```python
from build123d import *

# Parameters (mm, degrees)
EXTRUDE_1_DEPTH       = 2
SKETCH_2_R            = 1.6
CUT_EXTRUDE_1_DEPTH   = 2
CUT_EXTRUDE_2_DEPTH   = 10
EXTRUDE_START         = -2
EXTRUDE_1_2_OUTLINE_R = 16.5
EXTRUDE_1_2_DEPTH     = 2
SKETCH_5_R            = 1.6
CUT_EXTRUDE_3_DEPTH   = 2
FILLET_1_R            = 2
FILLET_2_R            = 2
SKETCH_6_W            = 33
SKETCH_6_H            = 4
EXTRUDE_2_DEPTH       = 2
FILLET_3_R            = 2


# Read off the part's stored shape, not the designer's step: 拉伸-薄壁1
with BuildPart() as part:
    # 草图1 → Extrude 1 (new body)
    with BuildSketch(Plane(origin=(0, 0, 0), x_dir=(1, 0, 0), z_dir=(0, 1, 0))):
        Polygon((0, 0), (121, 0), (121, -82), (-39.6, -82), (-39.6, 29), (0, 29), align=None)
    extrude(amount=EXTRUDE_1_DEPTH)

    # 草图2 → 切除-拉伸1 (cut)
    with BuildSketch(Plane(origin=(0, 2, 0), x_dir=(1, 0, 0), z_dir=(0, 1, 0))):
        with Locations(Location((-34.6, -75, 0), (0, 0, 270))):
            Circle(SKETCH_2_R)
        with Locations(Location((-34.6, 22, 0), (0, 0, 270))):
            Circle(SKETCH_2_R)
        with Locations(Location((116, -75, 0), (0, 0, 270))):
            Circle(SKETCH_2_R)
        with Locations(Location((116, -7, 0), (0, 0, 270))):
            Circle(SKETCH_2_R)
        with Locations(Location((5, -7, 0), (0, 0, 270))):
            Circle(SKETCH_2_R)
    extrude(amount=-CUT_EXTRUDE_1_DEPTH, mode=Mode.SUBTRACT)

    # 草图3 → 切除-拉伸2 (cut)
    with BuildSketch(Plane(origin=(0, 2, 0), x_dir=(1, 0, 0), z_dir=(0, 1, 0))):
        with BuildLine():
            Line((-8, 24), (-30.017424305, 24))
            ThreePointArc((-30.017424305, 24), (-30.162628331, 19.695714283), (-33.6, 17.101020514))
            Line((-33.6, 17.101020514), (-33.6, -70.101020514))
            ThreePointArc((-33.6, -70.101020514), (-30.428791604, -72.243005166), (-29.701020514, -76))
            Line((-29.701020514, -76), (-8, -76))
            Line((-8, -76), (-8, 24))
        make_face()
        with BuildLine():
            ThreePointArc((10, -7), (5, -12), (0, -7))
            Line((0, -7), (0, -75))
            Line((0, -75), (111, -75))
            ThreePointArc((111, -75), (111.527864045, -72.763932023), (113, -71))
            Line((113, -71), (113, -11))
            ThreePointArc((113, -11), (111.527864045, -9.236067977), (111, -7))
            Line((111, -7), (10, -7))
        make_face()
    extrude(amount=-CUT_EXTRUDE_2_DEPTH, mode=Mode.SUBTRACT)

    # Extrude 1 2 outline → Extrude 1 2 (add)
    # profile 1 of 4: a face of its own
    with BuildSketch(Plane(origin=(0, 2, 0), x_dir=(1, 0, 0), z_dir=(0, 1, 0)).offset(EXTRUDE_START)):
        with BuildLine():
            Line((87.508781443, -59.891378935), (111.047620543, -74.311568655))
            ThreePointArc((111.047620543, -74.311568655), (111.692830803, -72.460650968), (113, -71))
            Line((113, -71), (113, -70.81670339))
            Line((113, -70.81670339), (91.231047509, -57.480768531))
            Line((91.231047509, -57.480768531), (113, -43.382780251))
            Line((113, -43.382780251), (113, -38.617219749))
            Line((113, -38.617219749), (91.231047509, -24.519231469))
            Line((91.231047509, -24.519231469), (113, -11.18329661))
            Line((113, -11.18329661), (113, -11))
            ThreePointArc((113, -11), (111.692830803, -9.539349032), (111.047620543, -7.688431345))
            Line((111.047620543, -7.688431345), (87.508781443, -22.108621065))
            Line((87.508781443, -22.108621065), (64.179293034, -7))
            Line((64.179293034, -7), (56.417693677, -7))
            Line((56.417693677, -7), (31.597528439, -20.948522613))
            Line((31.597528439, -20.948522613), (9.952379457, -7.688431345))
            ThreePointArc((9.952379457, -7.688431345), (9.263558208, -9.611909533), (7.86285183, -11.099277912))
            Line((7.86285183, -11.099277912), (27.603885339, -23.192884025))
            Line((27.603885339, -23.192884025), (0, -38.705811323))
            Line((0, -38.705811323), (0, -43.294188677))
            Line((0, -43.294188677), (27.603885339, -58.807115975))
            Line((27.603885339, -58.807115975), (1.171383475, -75))
            Line((1.171383475, -75), (8.828616525, -75))
            Line((8.828616525, -75), (31.597528439, -61.051477387))
            Line((31.597528439, -61.051477387), (56.417693677, -75))
            Line((56.417693677, -75), (64.179293034, -75))
            Line((64.179293034, -75), (87.508781443, -59.891378935))
        make_face()
        with BuildLine():
            Line((35.503873282, -58.658401266), (44.147565445, -53.363166428))
            ThreePointArc((44.147565445, -53.363166428), (50.482041032, -58.885482887), (58.5, -61.402205763))
            Line((58.5, -61.402205763), (58.5, -71.581844381))
            Line((58.5, -71.581844381), (35.503873282, -58.658401266))
        make_face(mode=Mode.SUBTRACT)
        with BuildLine():
            Line((76.852434555, -53.363166428), (83.727285824, -57.574787025))
            Line((83.727285824, -57.574787025), (62.5, -71.321981654))
            Line((62.5, -71.321981654), (62.5, -61.402205763))
            ThreePointArc((62.5, -61.402205763), (70.517958968, -58.885482887), (76.852434555, -53.363166428))
        make_face(mode=Mode.SUBTRACT)
        with BuildLine():
            Line((31.510230182, -25.585960145), (42.058037819, -32.047680139))
            ThreePointArc((42.058037819, -32.047680139), (40, -41), (42.058037819, -49.952319861))
            Line((42.058037819, -49.952319861), (31.510230182, -56.414039855))
            Line((31.510230182, -56.414039855), (4.082306323, -41))
            Line((4.082306323, -41), (31.510230182, -25.585960145))
        make_face(mode=Mode.SUBTRACT)
        with BuildLine():
            Line((58.5, -10.418155619), (58.5, -20.597794237))
            ThreePointArc((58.5, -20.597794237), (50.482041032, -23.114517113), (44.147565445, -28.636833572))
            Line((44.147565445, -28.636833572), (35.503873282, -23.341598734))
            Line((35.503873282, -23.341598734), (58.5, -10.418155619))
        make_face(mode=Mode.SUBTRACT)
        with Locations((60.5, -41)):
            Circle(EXTRUDE_1_2_OUTLINE_R, mode=Mode.SUBTRACT)
        with BuildLine():
            Line((87.449551891, -26.83582338), (109.320706966, -41))
            Line((109.320706966, -41), (87.449551891, -55.16417662))
            Line((87.449551891, -55.16417662), (78.941962181, -49.952319861))
            ThreePointArc((78.941962181, -49.952319861), (81, -41), (78.941962181, -32.047680139))
            Line((78.941962181, -32.047680139), (87.449551891, -26.83582338))
        make_face(mode=Mode.SUBTRACT)
        with BuildLine():
            ThreePointArc((76.852434555, -28.636833572), (70.517958968, -23.114517113), (62.5, -20.597794237))
            Line((62.5, -20.597794237), (62.5, -10.678018346))
            Line((62.5, -10.678018346), (83.727285824, -24.425212975))
            Line((83.727285824, -24.425212975), (76.852434555, -28.636833572))
        make_face(mode=Mode.SUBTRACT)
    # profile 2 of 4: a face of its own
    with BuildSketch(Plane(origin=(0, 2, 0), x_dir=(1, 0, 0), z_dir=(0, 1, 0)).offset(EXTRUDE_START)):
        with BuildLine():
            Line((115.16418895, -76.364338627), (116.83581105, -73.635661373))
            ThreePointArc((116.83581105, -73.635661373), (114.635661373, -74.16418895), (115.16418895, -76.364338627))
        make_face()
    # profile 3 of 4: a face of its own
    with BuildSketch(Plane(origin=(0, 2, 0), x_dir=(1, 0, 0), z_dir=(0, 1, 0)).offset(EXTRUDE_START)):
        with BuildLine():
            Line((116.83581105, -8.364338627), (115.16418895, -5.635661373))
            ThreePointArc((115.16418895, -5.635661373), (114.635661373, -7.83581105), (116.83581105, -8.364338627))
        make_face()
    # profile 4 of 4: a face of its own
    with BuildSketch(Plane(origin=(0, 2, 0), x_dir=(1, 0, 0), z_dir=(0, 1, 0)).offset(EXTRUDE_START)):
        with BuildLine():
            Line((5.83581105, -5.635661373), (4.16418895, -8.364338627))
            ThreePointArc((4.16418895, -8.364338627), (6.364338627, -7.83581105), (5.83581105, -5.635661373))
        make_face()
    extrude(amount=EXTRUDE_1_2_DEPTH)

    # 草图5 → 切除-拉伸3 (cut)
    with BuildSketch(Plane(origin=(0, 2, 0), x_dir=(1, 0, 0), z_dir=(0, 1, 0))):
        with Locations(Location((116, -75, 0), (0, 0, 270))):
            Circle(SKETCH_5_R)
        with Locations(Location((116, -7, 0), (0, 0, 270))):
            Circle(SKETCH_5_R)
        with Locations(Location((5, -7, 0), (0, 0, 270))):
            Circle(SKETCH_5_R)
        Polygon((1.171383475, -75), (0, -75.717604291), (0, -75), align=None)
        Polygon((9.952379457, -7.688431345), (8.828616525, -7), (10, -7), (10.204957063, -7.513689319), align=None)
        Polygon((111, -7), (112.171383475, -7), (111.047620543, -7.688431345), (110.264993828, -7.459277871), align=None)
        Polygon((111.047620543, -74.311568655), (112.171383475, -75), (111, -75), (109.825525136, -74.655784327), align=None)
    extrude(amount=-CUT_EXTRUDE_3_DEPTH, mode=Mode.SUBTRACT)

    # 圆角1
    fillet_1_edges = [part.edges().sort_by_distance(p)[0] for p in [
        (0, 1, 38.705811323),
        (0, 1, 43.294188677),
        (8.828616525, 1, 75),
        (64.179293034, 1, 75),
        (56.417693677, 1, 75),
        (113, 1, 43.382780251),
        (113, 1, 38.617219749),
        (113, 1, 11.18329661),
        (113, 1, 70.81670339),
        (64.179293034, 1, 7),
        (56.417693677, 1, 7),
        (7.86285183, 1, 11.099277912),
        (31.597528439, 1, 61.051477387),
        (27.603885339, 1, 58.807115975),
        (27.603885339, 1, 23.192884025),
        (35.503873282, 1, 58.658401266),
        (35.503873282, 1, 23.341598734),
        (4.082306323, 1, 41),
        (31.597528439, 1, 20.948522613),
        (87.449551891, 1, 55.16417662),
        (109.320706966, 1, 41),
        (91.231047509, 1, 24.519231469),
        (91.231047509, 1, 57.480768531),
        (87.449551891, 1, 26.83582338),
        (78.941962181, 1, 49.952319861),
        (78.941962181, 1, 32.047680139),
        (76.852434555, 1, 53.363166428),
        (76.852434555, 1, 28.636833572),
        (87.508781443, 1, 22.108621065),
        (87.508781443, 1, 59.891378935),
        (62.5, 1, 20.597794237),
        (62.5, 1, 61.402205763),
        (83.727285824, 1, 57.574787025),
        (83.727285824, 1, 24.425212975),
        (44.147565445, 1, 53.363166428),
        (62.5, 1, 71.321981654),
        (58.5, 1, 71.581844381),
        (58.5, 1, 61.402205763),
        (31.510230182, 1, 56.414039855),
        (42.058037819, 1, 49.952319861),
        (44.147565445, 1, 28.636833572),
        (62.5, 1, 10.678018346),
        (58.5, 1, 10.418155619),
        (58.5, 1, 20.597794237),
        (31.510230182, 1, 25.585960145),
        (42.058037819, 1, 32.047680139),
        (0, 1, 75.717604291),
        (112.171383475, 1, 75),
        (112.171383475, 1, 7),
        (8.828616525, 1, 7),
        (-29.701020514, 1, 76),
        (-33.6, 1, 70.101020514),
        (-33.6, 1, -17.101020514),
        (-30.017424305, 1, -24),
        (-8, 1, -24),
        (-8, 1, 76),
        (0, 1, 7),
    ]]
    fillet(fillet_1_edges, radius=FILLET_1_R)

    # 圆角2
    fillet_2_edges = [part.edges().sort_by_distance(p)[0] for p in [
        (0, 1, 0),
        (121, 1, 0),
        (121, 1, 82),
        (-39.6, 1, 82),
        (-39.6, 1, -29),
        (0, 1, -29),
    ]]
    fillet(fillet_2_edges, radius=FILLET_2_R)

    # 草图6 → 拉伸-薄壁2 (add)
    with BuildSketch(Plane(origin=(0, 2, 0), x_dir=(1, 0, 0), z_dir=(0, 1, 0))):
        with Locations((60.5, -41)):
            Rectangle(SKETCH_6_W, SKETCH_6_H)
    extrude(amount=-EXTRUDE_2_DEPTH)

    # 圆角3
    fillet_3_edges = [part.edges().sort_by_distance(p)[0] for p in [
        (44.121660646, 1, 39),
        (76.878339354, 1, 39),
        (44.121660646, 1, 43),
        (76.878339354, 1, 43),
    ]]
    fillet(fillet_3_edges, radius=FILLET_3_R)


solid = part.part
```
Work out the finished part from the listing and answer in its coordinate system (mm). Round coordinates to 2 decimals unless told otherwise and drop trailing zeros. Write each loop counter-clockwise with the first axis right and the second up, starting at its lowest first coordinate (ties: lowest second). Pieces come first, ordered by that corner, then holes.
1) A cutting plane is placed at A-A on x = -16. Determine the outline of the cut face in (y, z), and give its area (3 significant figures).
2) Determine the mould class of faces 1 (the face through (40.3, 2, 42.7)), 2 (the face through (36.6, 0.986, 53.296)) for opening direction Z: pulls with the +Z half, pulls with the -Z half, needs draft (parallel to the pull), parting line crosses it, or undercut.
3) A cutting plane is placed at C-C on y = 0.6. Give the number of separate pieces and of enclosed holes in the cut face, and give its area (3 significant figures).
4) Flat-ended cylindrical pins translate along their axes: P1, Ø4, axis at x = -34.6, z = 75, coming from the +Y side; P2, Ø1, axis at x = 54.5, y = 1.5, coming from the -Z side. Find the tip coordinate at first contact, or state that the pin passes through.
5) A cutting plane is placed at B-B on x = 103. Determine the outline of the cut face in (y, z).
6) Consider probe 1 along Z at (x, y) = (116, 0.75); probe 2 along Z at (x, y) = (52, 0.4); probe 3 along Z at (x, y) = (-12.5, 1.95). Determine where each line is inside the solid, lowest interval first.
Entries:
1. outline: (0, -29) - (2, -29) - (2, -24) - (0, -24) - close; (0, 76) - (2, 76) - (2, 82) - (0, 82) - close
1. area: 22.0 mm2
2. face 1: needs draft
2. face 2: undercut
3. separate pieces: 1
3. enclosed holes: 22
3. area: 6,560 mm2
4. P1: stops at y = 2
4. P2: stops at z = 0
5. outline: (0, 0) - (2, 0) - (2, 7) - (0, 7) - close; (0, 12.62) - (2, 12.62) - (2, 17.31) - (0, 17.31) - close; (0, 32.14) - (2, 32.14) - (2, 36.91) - (0, 36.91) - close; (0, 45.09) - (2, 45.09) - (2, 49.86) - (0, 49.86) - close; (0, 64.69) - (2, 64.69) - (2, 69.38) - (0, 69.38) - close; (0, 75) - (2, 75) - (2, 82) - (0, 82) - close
6. probe 1: z = 0 to 5.4, 8.6 to 73.4, 76.6 to 82
6. probe 2: z = 0 to 14.07, 22.35 to 26.86, 39 to 43, 55.14 to 59.65, 67.93 to 82
6. probe 3: z = -29 to -24, 76 to 82
